```python
from build123d import *

# Parameters (mm, degrees)
F1_DEPTH = 6
F2_SIZE  = 5.99999
F3_R     = 1.5
F4_DEPTH = 6


# Not quite as in the source:
# - a fillet or chamfer is up to 0.001 mm smaller than in the source, because OpenCascade refuses the exact size


with BuildPart() as f1:
    # F0 (on Top) → F1 (new body)
    with BuildSketch(Plane.XY):
        Polygon((23.7662842423, 6.9127185345), (-3.7337157577, 6.9127185345), (-3.7337157577, -10.0872814655), (23.7662842423, -14.0872814655), align=None)
    extrude(amount=F1_DEPTH)

    # F2 (size 6 in the source; OpenCascade refuses exactly that, so slightly less here)
    f2_edges = [f1.edges().sort_by_distance(p)[0] for p in [
        (10.016284, -12.087281, 0),
    ]]
    chamfer(f2_edges, length=F2_SIZE)

    # F3 (on face) → F4 (cut, through all)
    with BuildSketch(Plane.XY.offset(6)):
        with Locations((0.0162842423, 0.9127185345)):
            Circle(F3_R)
        with Locations((10.0162842423, -1.5872814655)):
            Circle(F3_R)
        with Locations((20.0162842423, 0.9127185345)):
            Circle(F3_R)
    extrude(amount=-F4_DEPTH, mode=Mode.SUBTRACT)


solid = f1.part
```
Could you check a few things on this model? Use its own coordinates, in mm. Round coordinates to 2 decimals unless told otherwise and drop trailing zeros. Loops run counter-clockwise (first coordinate to the right, second up) from the corner with the lowest first, then second, coordinate; pieces in that order, holes last.
Q1. Please list where these lines run through material, in increasing order: L1, parallel to X at y = -0.25, z = 3.9; L2, parallel to Y at x = 10.25, z = 0.45; L3, parallel to Y at x = 20.75, z = 1.5.
Q2. I want a section at A-A (y = 0.25). Write out the boundary of the cut face in (x, z), and give its area (3 significant figures).
Q3. Thinking about a two-plate mould opening in X: for faces 1 (the cylindrical face through (8.518, -1.521, 3.042)), 2 (the flat face through (9.824, -8.985, 2.958)), 3 (the flat face through (23.766, -1, 3)), 4 (the flat face through (10, 6.913, 3)), which applies, pulls with the +X half, pulls with the -X half, needs draft (parallel to the pull), parting line crosses it, or undercut?
Q4. I want a section at B-B (z = 3.8). Write out the boundary of the cut face in (x, y), and give its area (3 significant figures).
Answer below:
1. L1: x = -3.73 to -0.93, 0.96 to 9.34, 10.7 to 19.07, 20.96 to 23.77
1. L2: y = -6.51 to -3.07, -0.11 to 6.91
1. L3: y = -9.1 to -0.4, 2.22 to 6.91
2. outline: (-3.73, 0) - (-1.33, 0) - (-1.33, 6) - (-3.73, 6) - close; (1.36, 0) - (18.67, 0) - (18.67, 6) - (1.36, 6) - close; (21.36, 0) - (23.77, 0) - (23.77, 6) - (21.36, 6) - close
2. area: 133 mm2
3. face 1: undercut
3. face 2: pulls with the -X half
3. face 3: pulls with the +X half
3. face 4: needs draft
4. outline: (-3.73, -7.86) - (23.77, -11.86) - (23.77, 6.91) - (-3.73, 6.91) - close; hole circle Ø3 at (0.02, 0.91); hole circle Ø3 at (10.02, -1.59); hole circle Ø3 at (20.02, 0.91)
4. area: 440 mm2
